For this review, take the finished solid that the model builds, in its own axes (mm). Face numbers are marked on the shaded views. A direction names the side the tool comes from. Give positions to 0.01 mm unless a question says otherwise; leave off trailing zeros. Order: outer loops, then holes, each group sorted by start corner. A loop starts at its lowest first (then second) coordinate and runs counter-clockwise, first axis right, second up. Notation, with made-up numbers: (88, 19.5) -> (144, 19.5) arc R27 ccw to (144, 57.5) -> close; hole circle Ø10 at (22, -1.75). An arc over 180 degrees is marked (long way). Return JSON: item names as keys, results as strings. Group by question number.
1) To check wall thickness, follow line 1 along X through (y, z) = (342.9, -594.75); line 2 along Y through (x, z) = (774.7, -592.25); line 3 along X through (y, z) = (342, -522). State the ranges of each line that lie inside material, in increasing order.
2) Add section A-A (y = 39). Give the boundary of the cut face in (x, z), then the cut area to 3 significant figures.
3) Add section C-C (z = -417). Give the boundary of the cut face in (x, y), then the cut area to 3 significant figures.
4) Add section B-B (x = 452.5). Give the boundary of the cut face in (y, z).
5) For the marked faces 1 and 2, list the 3-axis set-ups (+Z, -Z, +X, -X, +Y, -Y) from which the entire face can be reached by the end or side of a thin tool; tool diameter is ignored.
6) Insertion check: P1, Ø5, axis at x = 779.5, z = -524, coming from the -Y side; P2, Ø1.9, axis at x = 778, z = -595.5, coming from the +Y side; P3, Ø15, axis at x = -12.7, y = 342.9, coming from the +Z side. Each pin has a flat end and moves straight along its axis. Give the tip position at first contact, or say it passes through.
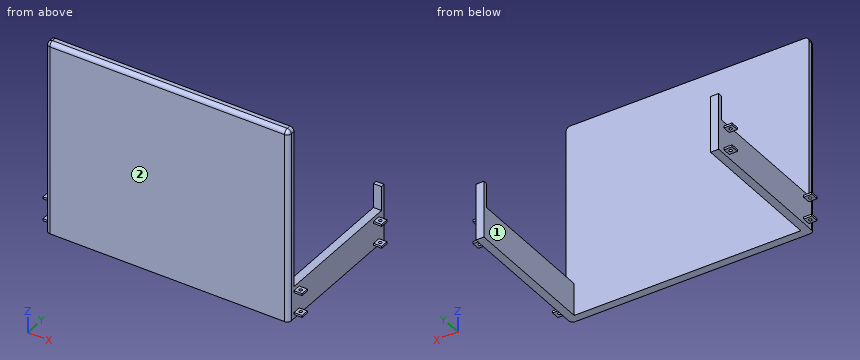
from build123d import *

# Parameters (mm, degrees)
SKETCH1_W                                      = 762
SKETCH1_H                                      = 381
BASE_STRUCTURE_DEPTH                           = 609.6
SKETCH3_W                                      = 711.2
SKETCH3_H                                      = 330.2
SHELL_CUT_DEPTH                                = 584.2
SKETCH5_W                                      = 25.4
SKETCH5_H                                      = 25.4
SKETCH5_R                                      = 4.7625
STABILITY_HOLDER_CUT_FOR_TOP_DEPTH             = 38.1
SKETCH7_W                                      = 63.5
SKETCH7_H                                      = 25.4
INSUDE_CUT_OF_STABILITY_HOLDERS_DEPTH          = 25.4
SKETCH14_W                                     = 711.2
SKETCH14_H                                     = 25.4
TOP_SHELLING_DEPTH                             = 406.4
SKETCH16_W                                     = 711.2
SKETCH16_H                                     = 50.8
BOTTOM_EXTENSION_DEPTH                         = 609.6
SKETCH16_6_W                                   = 711.2
SKETCH16_6_H                                   = 25.4
SKETCH16_6_H_2                                 = 50.8
BOTTOM_SHELLING_DEPTH                          = 584.2
SKETCH17_W                                     = 63.5
SKETCH17_H                                     = 25.4
BOTTOM_STABILTY_HOLDER_SHELL_CUT_DEPTH         = 25.4
SKETCH18_W                                     = 508
SKETCH18_H                                     = 406.4
F_3_4SHELL_FRONT_CHASSIS_CUT_DEPTH             = 763
FILLET_CORNER_OF_FRONT_CHASSIS_R               = 12.7
SKETCH95_W                                     = 508
SKETCH95_H                                     = 25.4
CUT_TOP_EXTRUSION_OF_CHASSIS_DEPTH             = 763
SKETCH171_W                                    = 76.290149759
SKETCH171_H                                    = 12.7
EXTRUSION_OF_STEERING_RACK_HOLDER_DEPTH        = 25.4
SKETCH172_W                                    = 76.2
SKETCH172_H                                    = 12.7
EXTRUSION_OF_OTHER_STEERING_RACK_HOLDER_DEPTH  = 25.4
MIRRORS_STABILITY_HOLDERS_COPY_1_SKETCH_W      = 25.4
MIRRORS_STABILITY_HOLDERS_COPY_1_SKETCH_H      = 25.4
MIRRORS_STABILITY_HOLDERS_COPY_1_SKETCH_R      = 4.7625
MIRRORS_STABILITY_HOLDERS_COPY_1_DEPTH         = 38.1
SKETCH173_W                                    = 63.5
SKETCH173_H                                    = 406.4
EXTRUSION_OF_OTHER_STABILITY_HOLDERS_TOP_DEPTH = 25.4
FILLET_OF_RIGHT_CORNER_OF_FRONT_CHASSIS_R      = 12.7
FILLET_OF_BOTTOM_SIDE_OF_FRONT_CHASSIS_R       = 12.7


with BuildPart() as part:
    # Sketch1 → Base Structure (new body)
    with BuildSketch(Plane.XY):
        with Locations((381, 190.5)):
            Rectangle(SKETCH1_W, SKETCH1_H)
    extrude(amount=-BASE_STRUCTURE_DEPTH)

    # Sketch3 → Shell Cut (cut)
    with BuildSketch(Plane(origin=(0, 0, -609.6), x_dir=(-1, 0, 0), z_dir=(0, 0, -1))):
        with Locations((-381, 190.5)):
            Rectangle(SKETCH3_W, SKETCH3_H)
    extrude(amount=-SHELL_CUT_DEPTH, mode=Mode.SUBTRACT)

    # Sketch5 → Stability Holder Cut for Top (add, symmetric)
    with BuildSketch(Plane.XY.offset(-558.8)):
        with Locations((774.7, 342.9)):
            Rectangle(SKETCH5_W, SKETCH5_H)
        with Locations((774.7, 342.9)):
            Circle(SKETCH5_R, mode=Mode.SUBTRACT)
    stability_holder_cut_for_top = extrude(amount=STABILITY_HOLDER_CUT_FOR_TOP_DEPTH, both=True)

    # Sketch7 → Insude Cut of Stability Holders (cut)
    with BuildSketch(Plane(origin=(787.4, 0, 0), x_dir=(0, 0, -1), z_dir=(1, 0, 0))):
        with Locations((558.8, 342.9)):
            Rectangle(SKETCH7_W, SKETCH7_H)
    extrude(amount=-INSUDE_CUT_OF_STABILITY_HOLDERS_DEPTH, mode=Mode.SUBTRACT)

    # Sketch14 → Top Shelling (cut)
    with BuildSketch(Plane(origin=(0, 0, -609.6), x_dir=(-1, 0, 0), z_dir=(0, 0, -1))):
        with Locations((-381, 368.3)):
            Rectangle(SKETCH14_W, SKETCH14_H)
    extrude(amount=-TOP_SHELLING_DEPTH, mode=Mode.SUBTRACT)

    # Sketch16 → Bottom Extension (add)
    with BuildSketch(Plane(origin=(0, 0, -609.6), x_dir=(-1, 0, 0), z_dir=(0, 0, -1))):
        Polygon((-736.6, -50.8), (-736.6, 0), (-762, 0), (-762, -76.2), (0, -76.2), (0, 0), (-25.4, 0), (-25.4, -50.8), align=None)
        with Locations((-381, -25.4)):
            Rectangle(SKETCH16_W, SKETCH16_H)
    extrude(amount=-BOTTOM_EXTENSION_DEPTH)

    # Sketch16<6> → Bottom Shelling (cut)
    with BuildSketch(Plane(origin=(0, 0, -609.6), x_dir=(-1, 0, 0), z_dir=(0, 0, -1))):
        with Locations((-381, 12.7)):
            Rectangle(SKETCH16_6_W, SKETCH16_6_H)
        with Locations((-381, -25.4)):
            Rectangle(SKETCH16_6_W, SKETCH16_6_H_2)
    extrude(amount=-BOTTOM_SHELLING_DEPTH, mode=Mode.SUBTRACT)

    # Mirror5: Stability Holder Cut for Top across plane
    add(stability_holder_cut_for_top.mirror(Plane.ZX.offset(152.4)))

    # Sketch17 → Bottom Stabilty Holder Shell Cut (cut)
    with BuildSketch(Plane(origin=(787.4, 0, 0), x_dir=(0, 0, -1), z_dir=(1, 0, 0))):
        with Locations((558.8, -38.1)):
            Rectangle(SKETCH17_W, SKETCH17_H)
    extrude(amount=-BOTTOM_STABILTY_HOLDER_SHELL_CUT_DEPTH, mode=Mode.SUBTRACT)

    # Sketch18 → 3/4Shell Front Chassis Cut (cut, through all)
    with BuildSketch(Plane(origin=(762, 0, 0), x_dir=(0, 0, -1), z_dir=(1, 0, 0))):
        with Locations((254, 152.4)):
            Rectangle(SKETCH18_W, SKETCH18_H)
    extrude(amount=-F_3_4SHELL_FRONT_CHASSIS_CUT_DEPTH, mode=Mode.SUBTRACT)

    # Fillet Corner of Front Chassis
    fillet_corner_of_front_chassis_edges = [part.edges().sort_by_distance(p)[0] for p in [
        (762, -63.5, 0),
    ]]
    fillet(fillet_corner_of_front_chassis_edges, radius=FILLET_CORNER_OF_FRONT_CHASSIS_R)

    # Sketch95 → Cut Top Extrusion of Chassis (cut, through all)
    with BuildSketch(Plane(origin=(762, 0, 0), x_dir=(0, 0, -1), z_dir=(1, 0, 0))):
        with Locations((254, 368.3)):
            Rectangle(SKETCH95_W, SKETCH95_H)
    extrude(amount=-CUT_TOP_EXTRUSION_OF_CHASSIS_DEPTH, mode=Mode.SUBTRACT)

    # Sketch171 → Extrusion of Steering Rack Holder (add)
    with BuildSketch(Plane(origin=(762, 0, 0), x_dir=(0, 0, -1), z_dir=(1, 0, 0))):
        with Locations((469.854925121, 374.65)):
            Rectangle(SKETCH171_W, SKETCH171_H)
    extrude(amount=-EXTRUSION_OF_STEERING_RACK_HOLDER_DEPTH)

    # Sketch172 → Extrusion of Other Steering Rack Holder (add)
    with BuildSketch(Plane.ZY):
        with Locations((-469.9, 374.65)):
            Rectangle(SKETCH172_W, SKETCH172_H)
    extrude(amount=-EXTRUSION_OF_OTHER_STEERING_RACK_HOLDER_DEPTH)

    # Mirrors Stability Holders: Stability Holder Cut for Top across plane
    add(stability_holder_cut_for_top.mirror(Plane(origin=(381, 0, 0), x_dir=(0, 0, 1), z_dir=(1, 0, 0))))

    # Mirrors Stability Holders copy 1 sketch → Mirrors Stability Holders copy 1 (add, symmetric)
    with BuildSketch(Plane(origin=(762, 304.8, -558.8), x_dir=(-1, 0, 0), z_dir=(0, 0, 1))):
        with Locations((774.7, 342.9)):
            Rectangle(MIRRORS_STABILITY_HOLDERS_COPY_1_SKETCH_W, MIRRORS_STABILITY_HOLDERS_COPY_1_SKETCH_H)
        with Locations((774.7, 342.9)):
            Circle(MIRRORS_STABILITY_HOLDERS_COPY_1_SKETCH_R, mode=Mode.SUBTRACT)
    extrude(amount=MIRRORS_STABILITY_HOLDERS_COPY_1_DEPTH, both=True)

    # Sketch173 → Extrusion of Other Stability Holders Top and Bottom (cut)
    with BuildSketch(Plane.ZY.offset(25.4)):
        with Locations((-558.8, 152.4)):
            Rectangle(SKETCH173_W, SKETCH173_H)
    extrude(amount=-EXTRUSION_OF_OTHER_STABILITY_HOLDERS_TOP_DEPTH, mode=Mode.SUBTRACT)

    # Fillet of Right Corner of Front Chassis
    fillet_of_right_corner_of_front_chassis_edges = [part.edges().sort_by_distance(p)[0] for p in [
        (0, -63.5, 0),
    ]]
    fillet(fillet_of_right_corner_of_front_chassis_edges, radius=FILLET_OF_RIGHT_CORNER_OF_FRONT_CHASSIS_R)

    # Fillet of Bottom Side of Front Chassis
    fillet_of_bottom_side_of_front_chassis_edges = [part.edges().sort_by_distance(p)[0] for p in [
        (381, -76.2, 0),
        (762, -76.2, -311.15),
        (758.280256121, -76.2, -3.719743879),
        (0, -76.2, -311.15),
        (3.719743879, -76.2, -3.719743879),
    ]]
    fillet(fillet_of_bottom_side_of_front_chassis_edges, radius=FILLET_OF_BOTTOM_SIDE_OF_FRONT_CHASSIS_R)


solid = part.part
Evaluation:
{
 "1": {"line 1": "-25.4 to -17.46, -7.94 to 25.4, 736.6 to 769.94, 779.46 to 787.4", "line 2": "-50.8 to -42.86, -33.34 to -25.4, 330.2 to 338.14, 347.66 to 355.6", "line 3": "-25.4 to -17.38, -8.02 to 25.4, 736.6 to 770.02, 779.38 to 787.4"},
 "2": {"outline": "(0, -609.6) -> (25.4, -609.6) -> (25.4, -508) -> (0, -508) -> close; (736.6, -609.6) -> (762, -609.6) -> (762, -508) -> (736.6, -508) -> close", "area": "5,160 mm^2"},
 "3": {"outline": "(0, -63.5) arc R12.7 ccw to (12.7, -76.2) -> (749.3, -76.2) arc R12.7 ccw to (762, -63.5) -> (762, -50.8) -> (0, -50.8) -> close", "area": "19,300 mm^2"},
 "4": {"outline": "(-76.2, -609.6) -> (-50.8, -609.6) -> (-50.8, 0) -> (-63.5, 0) arc R12.7 ccw to (-76.2, -12.7) -> close"},
 "5": {"face 1": "+Z, -Z, +Y", "face 2": "+Z, -Z, +X, -X, -Y"},
 "6": {"P1": "y = -50.8", "P2": "y = 355.6", "P3": "z = -520.7"}
}
